Part model, mm, in its own coordinate system. A direction names the side the tool comes from. Round coordinates to 2 decimals unless told otherwise and drop trailing zeros. Write each loop counter-clockwise with the first axis right and the second up, starting at its lowest first coordinate (ties: lowest second). Pieces come first, ordered by that corner, then holes.
1) Saw through at B-B on z = 6.6. Write the cut outline in (x, y), and give its area (3 significant figures).
2) Flat gauge pins, fed straight in: pin 1 (1.4 mm diameter, centred on x = -28.5, z = 12, fed in from -Y); pin 2 (3 mm diameter, centred on x = -28, z = -13, fed in from -Y); pin 3 (4.5 mm diameter, centred on x = 44.5, z = 30, fed in from -Y). Where does each tip first touch, or does it go through?
3) Drill centre lines: L1, parallel to X at y = -30, z = -33.7; L2, parallel to X at y = -51.25, z = -30; L3, parallel to X at y = -30.5, z = 30. Where is each one in solid material? Low to high.
4) Which spindle directions (+Z, -Z, +X, -X, +Y, -Y) get a long thin tool onto all of the face, cutting with end or side? Do faces 3 (the flat face through (19.028, -27.535, -30.535)), 4 (the flat face through (27.729, -32.465, -30.535)), 5 (the cylindrical face through (-41.92, -2.03, 5.86)). Say none if no direction does.
5) Pull direction X, two halves, no side cores. Call faces 1 (the flat face through (-50, -27, 0)), 2 (the flat face through (-47, -29, -24.9)): +X half, -X half, draft (parallel to the pull), parting line (faces both ways), or undercut.
6) Saw through at A-A on y = -7. Count the separate pieces of the cut face and the enclosed holes in it, and give its area (3 significant figures).
7) Saw through at D-D on x = 33. Write the cut outline in (y, z), and give its area (3 significant figures).
8) Saw through at C-C on y = -23. Write the cut outline in (x, z), and give its area (3 significant figures).
```python
from build123d import *

# Parameters (mm, degrees)
SKIZZE1_W                       = 100
SKIZZE1_H                       = 70
AUFSATZ_LINEAR_AUSTRAGEN1_DEPTH = 4
SKIZZE2_W                       = 100
SKIZZE2_H                       = 70
SKIZZE2_R                       = 2.1
AUFSATZ_LINEAR_AUSTRAGEN2_DEPTH = 50
SKIZZE3_R                       = 2.8
SCHNITT_LINEAR_AUSTRAGEN1_DEPTH = 9
SCHNITT_LINEAR_AUSTRAGEN3_REACH = 80.899
SKIZZE5_R                       = 1.6
SKIZZE6_R                       = 2.1
SKIZZE6_W                       = 20
SKIZZE6_H                       = 15
SCHNITT_LINEAR_AUSTRAGEN4_DEPTH = 2
AUFSATZ_LINEAR_AUSTRAGEN3_DEPTH = 5
SKETCH2_R                       = 3.95
SKETCH2_R_2                     = 1.45
BOSS_EXTRUDE1_DEPTH             = 5


with BuildPart() as part:
    # Skizze1 → Aufsatz-Linear austragen1 (new body)
    with BuildSketch(Plane.XZ):
        Rectangle(SKIZZE1_W, SKIZZE1_H)
    extrude(amount=AUFSATZ_LINEAR_AUSTRAGEN1_DEPTH)

    # Skizze2 → Aufsatz-Linear austragen2 (add)
    with BuildSketch(Plane.XZ.offset(4)):
        Rectangle(SKIZZE2_W, SKIZZE2_H)
        with Locations(Location((-45, 30, 0), (0, 0, 270))):
            Circle(SKIZZE2_R, mode=Mode.SUBTRACT)
        with Locations(Location((45, 30, 0), (0, 0, 90))):
            Circle(SKIZZE2_R, mode=Mode.SUBTRACT)
        with Locations(Location((45, -30, 0), (0, 0, 270))):
            Circle(SKIZZE2_R, mode=Mode.SUBTRACT)
        with Locations(Location((-45, -30, 0), (0, 0, 90))):
            Circle(SKIZZE2_R, mode=Mode.SUBTRACT)
        with BuildLine():
            Line((-48, 24.9), (-48, -24.9))
            Line((-48, -24.9), (-45, -24.9))
            ThreePointArc((-45, -24.9), (-41.393755416, -26.393755416), (-39.9, -30))
            Line((-39.9, -30), (-39.9, -33))
            Line((-39.9, -33), (39.9, -33))
            Line((39.9, -33), (39.9, -30))
            ThreePointArc((39.9, -30), (41.393755416, -26.393755416), (45, -24.9))
            Line((45, -24.9), (48, -24.9))
            Line((48, -24.9), (48, 24.9))
            Line((48, 24.9), (45, 24.9))
            ThreePointArc((45, 24.9), (41.393755416, 26.393755416), (39.9, 30))
            Line((39.9, 30), (39.9, 33))
            Line((39.9, 33), (-39.9, 33))
            Line((-39.9, 33), (-39.9, 30))
            ThreePointArc((-39.9, 30), (-41.393755416, 26.393755416), (-45, 24.9))
            Line((-45, 24.9), (-48, 24.9))
        make_face(mode=Mode.SUBTRACT)
    extrude(amount=AUFSATZ_LINEAR_AUSTRAGEN2_DEPTH)

    # Skizze3 → Schnitt-Linear austragen1 (cut)
    with BuildSketch(Plane.XZ.offset(54)):
        with Locations(Location((-45, 30, 0), (0, 0, 270))):
            Circle(SKIZZE3_R)
        with Locations(Location((45, 30, 0), (0, 0, 90))):
            Circle(SKIZZE3_R)
        with Locations(Location((45, -30, 0), (0, 0, 270))):
            Circle(SKIZZE3_R)
        with Locations(Location((-45, -30, 0), (0, 0, 90))):
            Circle(SKIZZE3_R)
    extrude(amount=-SCHNITT_LINEAR_AUSTRAGEN1_DEPTH, mode=Mode.SUBTRACT)

    # Skizze5 → Schnitt-Linear austragen3 (cut, up to next)
    with BuildSketch(Plane.XZ.offset(4), mode=Mode.PRIVATE) as schnitt_linear_austragen3_sk1:
        with Locations(Location((-40.5, 6.6, 0), (0, 0, 270))):
            Circle(SKIZZE5_R)
    schnitt_linear_austragen3_tool1 = extrude(schnitt_linear_austragen3_sk1.sketch, amount=-SCHNITT_LINEAR_AUSTRAGEN3_REACH, mode=Mode.PRIVATE) & part.part
    # Skizze5 → Schnitt-Linear austragen3 (cut, up to next)
    with BuildSketch(Plane.XZ.offset(4), mode=Mode.PRIVATE) as schnitt_linear_austragen3_sk2:
        with Locations(Location((-40.5, -6.6, 0), (0, 0, 90))):
            Circle(SKIZZE5_R)
    schnitt_linear_austragen3_tool2 = extrude(schnitt_linear_austragen3_sk2.sketch, amount=-SCHNITT_LINEAR_AUSTRAGEN3_REACH, mode=Mode.PRIVATE) & part.part
    add(schnitt_linear_austragen3_tool1.solids().sort_by_distance((-40.5, -4, 6.6))[0], mode=Mode.SUBTRACT)
    add(schnitt_linear_austragen3_tool2.solids().sort_by_distance((-40.5, -4, -6.6))[0], mode=Mode.SUBTRACT)

    # Skizze6 → Schnitt-Linear austragen4 (cut)
    with BuildSketch(Plane(origin=(0, 0, -35), x_dir=(1, 0, 0), z_dir=(0, 0, -1))):
        with Locations(Location((-23.378367252, 30, 0), (0, 0, 270))):
            Circle(SKIZZE6_R)
        with Locations((23.378367252, 30)):
            Circle(SKIZZE6_R)
        with Locations((25.02457838, 46.5)):
            Rectangle(SKIZZE6_W, SKIZZE6_H)
    extrude(amount=-SCHNITT_LINEAR_AUSTRAGEN4_DEPTH, mode=Mode.SUBTRACT)

    # Skizze7 → Aufsatz-Linear austragen3 (add)
    # profile 1 of 2: a face of its own
    with BuildSketch(Plane.XY.offset(-33)):
        Polygon((-17.604864561, -30), (-20.491615906, -25), (-26.265118598, -25), (-29.151869944, -30), (-26.265118598, -35), (-20.491615906, -35), align=None)
        Polygon((-19.336915368, -30), (-21.35764131, -26.5), (-25.399093195, -26.5), (-27.419819137, -30), (-25.399093195, -33.5), (-21.35764131, -33.5), align=None, mode=Mode.SUBTRACT)
    # profile 2 of 2: a face of its own
    with BuildSketch(Plane.XY.offset(-33)):
        Polygon((20.491615906, -35), (17.604864561, -30), (20.491615906, -25), (26.265118598, -25), (29.151869944, -30), (26.265118598, -35), align=None)
        Polygon((21.35764131, -33.5), (19.336915368, -30), (21.35764131, -26.5), (25.399093195, -26.5), (27.419819137, -30), (25.399093195, -33.5), align=None, mode=Mode.SUBTRACT)
    extrude(amount=AUFSATZ_LINEAR_AUSTRAGEN3_DEPTH)

    # Sketch2 → Boss-Extrude1 (add)
    # profile 1 of 4: a face of its own
    with BuildSketch(Plane.XZ.offset(4)):
        with Locations(Location((-28, -12.5, 0), (0, 0, 90))):
            Circle(SKETCH2_R)
        with Locations(Location((-28, -12.5, 0), (0, 0, 270))):
            Circle(SKETCH2_R_2, mode=Mode.SUBTRACT)
    # profile 2 of 4: a face of its own
    with BuildSketch(Plane.XZ.offset(4)):
        with Locations(Location((9, -16.5, 0), (0, 0, 90))):
            Circle(SKETCH2_R)
        with Locations(Location((9, -16.5, 0), (0, 0, 270))):
            Circle(SKETCH2_R_2, mode=Mode.SUBTRACT)
    # profile 3 of 4: a face of its own
    with BuildSketch(Plane.XZ.offset(4)):
        with Locations(Location((9, 16.5, 0), (0, 0, 90))):
            Circle(SKETCH2_R)
        with Locations(Location((9, 16.5, 0), (0, 0, 90))):
            Circle(SKETCH2_R_2, mode=Mode.SUBTRACT)
    # profile 4 of 4: a face of its own
    with BuildSketch(Plane.XZ.offset(4)):
        with Locations(Location((-28, 12.5, 0), (0, 0, 90))):
            Circle(SKETCH2_R)
        with Locations(Location((-28, 12.5, 0), (0, 0, 90))):
            Circle(SKETCH2_R_2, mode=Mode.SUBTRACT)
    extrude(amount=BOSS_EXTRUDE1_DEPTH)


solid = part.part
```
Completed:
1. outline: (-50, -54) - (-48, -54) - (-48, -4) - (-42.1, -4) - (-42.1, 0) - (-50, 0) - close; (-38.9, -4) - (48, -4) - (48, -54) - (50, -54) - (50, 0) - (-38.9, 0) - close
1. area: 587 mm2
2. pin 1: stops at y = -4
2. pin 2: stops at y = -9
2. pin 3: stops at y = -45
3. L1: x = -50 to -25.48, -21.28 to 21.28, 25.48 to 50
3. L2: x = -50 to -47.8, -42.2 to -39.9, 39.9 to 42.2, 47.8 to 50
3. L3: x = -50 to -47.1, -42.9 to -39.9, 39.9 to 42.9, 47.1 to 50
4. face 3: none
4. face 4: -Y
4. face 5: +Y, -Y
5. face 1: -X half
5. face 2: undercut
6. separate pieces: 5
6. enclosed holes: 9
6. area: 1,020 mm2
7. outline: (-54, 33) - (-4, 33) - (-4, -33) - (-39, -33) - (-39, -35) - (0, -35) - (0, 35) - (-54, 35) - close
7. area: 450 mm2
8. outline: (-50, -35) - (50, -35) - (50, 35) - (-50, 35) - close; hole (-48, -24.9) - (-45, -24.9) arc R5.1 cw to (-39.9, -30) - (-39.9, -33) - (39.9, -33) - (39.9, -30) arc R5.1 cw to (45, -24.9) - (48, -24.9) - (48, 24.9) - (45, 24.9) arc R5.1 cw to (39.9, 30) - (39.9, 33) - (-39.9, 33) - (-39.9, 30) arc R5.1 cw to (-45, 24.9) - (-48, 24.9) - close; hole circle Ø4.2 at (-45, -30); hole circle Ø4.2 at (-45, 30); hole circle Ø4.2 at (45, -30); hole circle Ø4.2 at (45, 30)
8. area: 849 mm2
